from build123d import *

# Parameters (mm, degrees)
BOSS_EXTRUDE1_DEPTH  = 3
M3_CLEARANCE_HOLE1_D = 3.4
FILLET1_R            = 1
CUT_EXTRUDE1_DEPTH   = 93.987352344
FILLET2_R            = 3


with BuildPart() as part:
    # Sketch1 → Boss-Extrude1 (new body)
    with BuildSketch(Plane.XY):
        with BuildLine():
            Line((-7.745, -8), (7.745, -8))
            Line((7.745, -8), (70.519857407, 20.746231418))
            ThreePointArc((70.519857407, 20.746231418), (73.107899278, 27.441010115), (66.482157687, 30.201004841))
            Line((66.482157687, 30.201004841), (53.337310845, 24.984396605))
            ThreePointArc((53.337310845, 24.984396605), (41.652152386, 30.029896758), (46.697652539, 41.715055217))
            Line((46.697652539, 41.715055217), (59.842499382, 46.931663453))
            ThreePointArc((59.842499382, 46.931663453), (62.807533315, 53.385795263), (56.49682568, 56.644968901))
            Line((56.49682568, 56.644968901), (29.473725399, 48.709154624))
            ThreePointArc((29.473725399, 48.709154624), (28.966294631, 48.540909296), (28.471678813, 48.338060414))
            Line((28.471678813, 48.338060414), (-3.1843478, 34.060095898))
            ThreePointArc((-3.1843478, 34.060095898), (-6.505682082, 31.202514205), (-7.745, 27))
            Line((-7.745, 27), (-7.745, -8))
        make_face()
    extrude(amount=BOSS_EXTRUDE1_DEPTH)

    # M3 Clearance Hole1 (through all)
    with Locations(Plane(origin=(0, 0, 0), x_dir=(1, 0, 0), z_dir=(0, 0, -1))):
        with Locations((57.945720298, -51.711180989), (68.378936771, -25.421487305), (42.089243086, -14.988270832), (31.656026613, -41.277964517), (0, -27), (0, 0)):
            Hole(M3_CLEARANCE_HOLE1_D / 2)

    # Fillet1
    fillet1_edges = [part.edges().sort_by_distance(p)[0] for p in [
        (7.745, -8, 1.5),
        (-7.745, -8, 1.5),
    ]]
    fillet(fillet1_edges, radius=FILLET1_R)

    # Sketch4 → Cut-Extrude1 (cut, through all)
    with BuildSketch(Plane(origin=(0, 0, 0), x_dir=(-1, 0, 0), z_dir=(0, 0, -1))):
        with BuildLine():
            ThreePointArc((-37.446464364, 17.198737867), (-37.2921785, 16.840223889), (-37.165529718, 16.471040349))
            Line((-37.165529718, 16.471040349), (-7.121534424, 2.713117557))
            Line((-7.121534424, 2.713117557), (-30.893579986, 33.710742913))
            Line((-30.893579986, 33.710742913), (-37.446464364, 17.198737867))
        make_face()
        with BuildLine():
            Line((-21.049163615, 34.020143008), (2.745, 2.993676756))
            Line((2.745, 2.993676756), (2.745, 22.820888252))
            ThreePointArc((2.745, 22.820888252), (-2.276587416, 22.548354266), (-4.995123002, 26.779214606))
            Line((-4.995123002, 26.779214606), (-21.049163615, 34.020143008))
        make_face()
    extrude(amount=-CUT_EXTRUDE1_DEPTH, mode=Mode.SUBTRACT)

    # Fillet2
    fillet2_edges = [part.edges().sort_by_distance(p)[0] for p in [
        (30.893579986, 33.710742913, 1.5),
        (7.121534424, 2.713117557, 1.5),
        (-2.745, 22.820888252, 1.5),
        (-2.745, 2.993676756, 1.5),
        (21.049163615, 34.020143008, 1.5),
        (4.995123002, 26.779214606, 1.5),
    ]]
    fillet(fillet2_edges, radius=FILLET2_R)


solid = part.part
Design review of the part built by this model. Coordinates are the model's own, in mm. A direction names the side the tool comes from. Round coordinates to 2 decimals unless told otherwise and drop trailing zeros. Write each loop counter-clockwise with the first axis right and the second up, starting at its lowest first coordinate (ties: lowest second). Pieces come first, ordered by that corner, then holes. Notation, with made-up numbers: (-13, 49.25) -> (31, 49.25) arc R19 cw to (31, 58.25) -> close; hole circle Ø1 at (29.25, 84). An arc over 180 degrees is marked (long way). One line per item, written item: value. Start each with the question number.
Q1. Insertion check: P1, Ø0.9, axis at y = 16.5, z = 1.5, coming from the +X side; P2, Ø4.5, axis at x = 68.38, y = 25.42, coming from the +Z side; P3, Ø1.5, axis at x = 41, z = 0.5, coming from the +Y side. Each pin has a flat end and moves straight along its axis. Give the tip position at first contact, or say it passes through.
Q2. Add section A-A (x = 20.5). Give the boundary of the cut face in (y, z), then the cut area to 3 significant figures.
Q3. Add section C-C (z = 1.2). State how many separate pieces and enclosed holes the cut face has, then the cut area to 3 significant figures.
Q4. The part is to be moulded in two halves that separate along X. For faces 3 (the face through (0.221, 25.314, 1.521)), 4 (the face through (-6.472, 31.255, 1.479)), 5 (the face through (23, 25, 3)), say which applies: pulls with the +X half, pulls with the -X half, needs draft (parallel to the pull), parting line crosses it, or undercut.
Q5. To check wall thickness, follow probe 1 along Y at (x, z) = (0.5, 2.2); probe 2 along Y at (x, z) = (0, 2.2); probe 3 along X at (y, z) = (20, 1.55) (3 decimals). State the ranges of each line that lie inside material, in increasing order.
Q6. Add section B-B (y = 0). Give the boundary of the cut face in (x, z) (3 decimals), then the cut area to 3 significant figures.
Q7. Add section D-D (x = 65). Give the boundary of the cut face in (y, z), then the cut area to 3 significant figures.
Q8. Tool access review of faces 1 (the face through (12.87, 41.3, 1.48)), 2 (the face through (60, 27.63, 1.48)): name each direction out of +Z, -Z, +X, -X, +Y, -Y from which nothing blocks a thin tool from reaching the whole face with its end or side.
Response:
1. P1: stops at x = 62.23
1. P2: stops at z = 3
1. P3: stops at y = 52.31
2. outline: (-2.16, 0) -> (8.84, 0) -> (8.84, 3) -> (-2.16, 3) -> close; (20.16, 0) -> (44.74, 0) -> (44.74, 3) -> (20.16, 3) -> close
2. area: 107 mm^2
3. separate pieces: 1
3. enclosed holes: 8
3. area: 2,360 mm^2
4. face 3: undercut
4. face 4: pulls with the -X half
4. face 5: needs draft
5. probe 1: y = -8 to -1.62, 1.62 to 8.85, 22.03 to 25.38, 28.62 to 35.72
5. probe 2: y = -8 to -1.7, 1.7 to 8.85, 21.99 to 25.3, 28.7 to 35.5
5. probe 3: x = -7.745 to -2.575, 10.297 to 20.379, 36.335 to 68.89
6. outline: (-7.745, 0) -> (-1.7, 0) -> (-1.7, 3) -> (-7.745, 3) -> close; (1.7, 0) -> (25.215, 0) -> (25.215, 3) -> (1.7, 3) -> close
6. area: 88.7 mm^2
7. outline: (18.22, 0) -> (29.61, 0) -> (29.61, 3) -> (18.22, 3) -> close
7. area: 34.2 mm^2
8. face 1: +Z, -Z, -X, +Y
8. face 2: +Z, -Z
